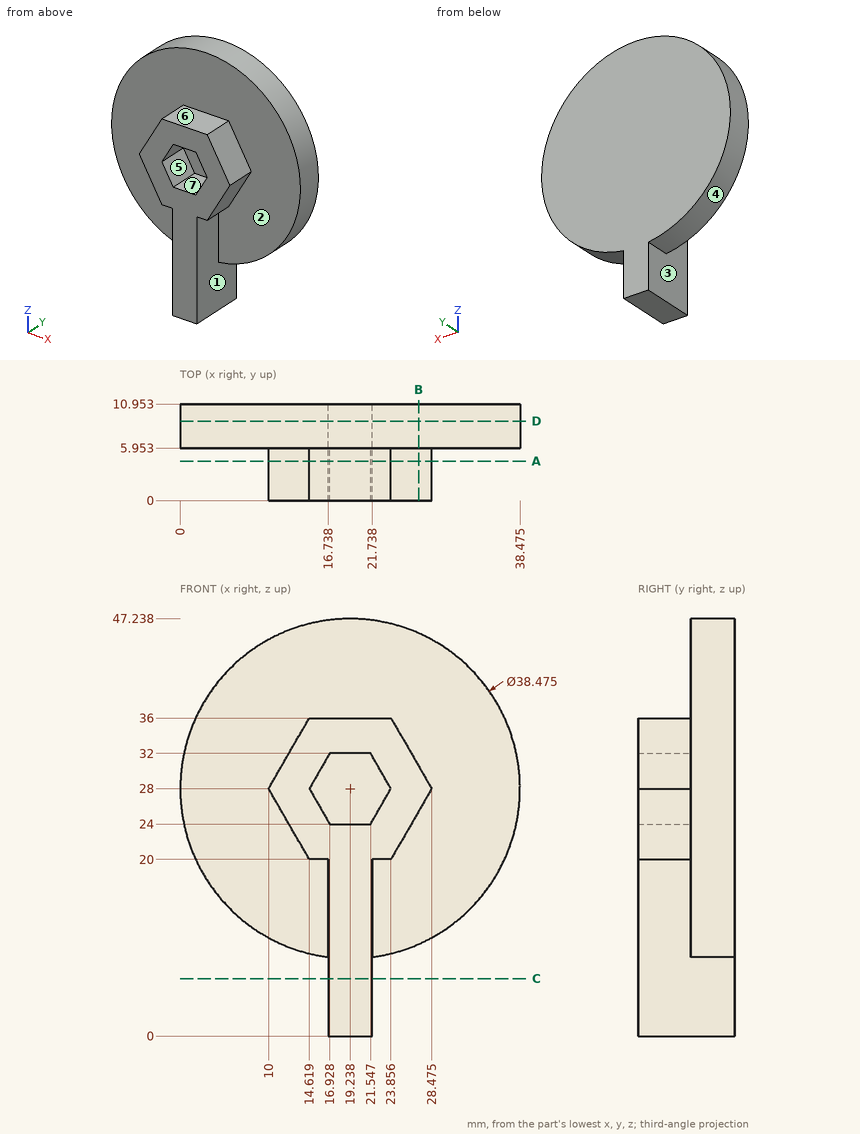
Job drawing, mm, ordinate dimensions from the low corner. One solid piece. A direction names the side the tool comes from. Give positions to 0.01 mm unless a question says otherwise; leave off trailing zeros. Order: outer loops, then holes, each group sorted by start corner. A loop starts at its lowest first (then second) coordinate and runs counter-clockwise, first axis right, second up. Notation, with made-up numbers: (83, 1.25) - (115, 1.25) arc R14 ccw to (115, 26.25) - close; hole circle Ø2 at (42, 85.5). An arc over 180 degrees is marked (long way). One line per question, with ' | ' between items.
1. Band-saw the part on D-D on y = 9. List the corners of the cut face in (x, z) (1 decimal), then the cut area to 3 significant figures.
Filled in:
outline: (16.7, 0) - (21.7, 0) - (21.7, 8.9) arc R19.2 ccw (long way) to (16.7, 8.9) - close | area: 1,210 mm²
2. Drill centre lines: probe 1 along X at (y, z) = (1, 28) (1 decimal); probe 2 along X at (y, z) = (3, 25.5) (1 decimal); probe 3 along X at (y, z) = (5.5, 12). Where is each one in solid material? Low to high.
Filled in:
probe 1: 10 to 14.6, 23.9 to 28.5 | probe 2: 11.4 to 16.1, 22.4 to 27 | probe 3: 16.74 to 21.74
3. Pull direction X, two halves, no side cores. Call the marked faces 4, 5, 6 and 7: +X half, -X half, draft (parallel to the pull), parting line (faces both ways), or undercut.
Filled in:
face 4: parting line | face 5: undercut | face 6: draft | face 7: undercut
4. Band-saw the part on B-B on x = 27. List the corners of the cut face in (y, z) (1 decimal).
Filled in:
outline: (0, 25.4) - (6, 25.4) - (6, 10.4) - (11, 10.4) - (11, 45.6) - (6, 45.6) - (6, 30.6) - (0, 30.6) - close
5. Which spindle directions (+Z, -Z, +X, -X, +Y, -Y) get a long thin tool onto all of the face, cutting with end or side? Do the marked faces 1, 2 and 3. Say none if no direction does.
Filled in:
face 1: -Z, +X, -Y | face 2: -Y | face 3: -Z, -X, -Y
6. Band-saw the part on C-C on z = 6.5. List the corners of the cut face in (x, y).
Filled in:
outline: (16.74, 0) - (21.74, 0) - (21.74, 10.95) - (16.74, 10.95) - close
7. Band-saw the part on A-A on y = 4.5. List the corners of the cut face in (x, z) (1 decimal).
Filled in:
outline: (10, 28) - (14.6, 20) - (16.7, 20) - (16.7, 0) - (21.7, 0) - (21.7, 20) - (23.9, 20) - (28.5, 28) - (23.9, 36) - (14.6, 36) - close; hole (14.6, 28) - (16.9, 24) - (21.5, 24) - (23.9, 28) - (21.5, 32) - (16.9, 32) - close
8. Drop flat-ended pins along their axis: P1, Ø2.5, axis at x = 19, y = 4, coming from the +Z side; P2, Ø2, axis at x = 23, y = 7.5, coming from the +Z side; P3, Ø1.7, axis at x = 23, y = 2.5, coming from the -Z side. Give the stop position or say it passes through.
Filled in:
P1: z = 36 | P2: z = 47.04 | P3: z = 20
